```python
from build123d import *

# Parameters (mm, degrees)
BOSS_EXTRUDE1_DEPTH      = 70
BOSS_EXTRUDE1_DEPTH_BACK = 70
SKETCH1_W                = 20
SKETCH1_H                = 10
SKETCH3_W                = 20
SKETCH3_H                = 5
BOSS_EXTRUDE2_DEPTH      = 20
FILLET1_R                = 10
SKETCH4_R                = 2.75
CUT_EXTRUDE1_DEPTH       = 91.863909227
FILLET1_OF_MIRROR1_R     = 10
CHAMFER1_SIZE            = 8.660254038
CHAMFER1_SIZE_2          = 5
SKETCH5_R                = 8.5
CUT_EXTRUDE2_DEPTH       = 5
CUT_EXTRUDE3_DEPTH       = 91.691785736
CUT_EXTRUDE3_DEPTH_BACK  = 91.691785736
SKETCH6_R                = 2


# Some blends are built 0.0001 mm under size
with BuildPart() as part:
    # Sketch1 → Boss-Extrude1 (new, two sides: drawn at the far end of the back side and taken through both)
    with BuildSketch(Plane.XY.offset(-BOSS_EXTRUDE1_DEPTH_BACK)):
        Rectangle(SKETCH1_W, SKETCH1_H)
    extrude(amount=BOSS_EXTRUDE1_DEPTH + BOSS_EXTRUDE1_DEPTH_BACK)

    # Sketch3 → Boss-Extrude2 (add)
    with BuildSketch(Plane(origin=(0, 0, -70), x_dir=(-1, 0, 0), z_dir=(0, 0, -1))):
        Rectangle(SKETCH3_W, SKETCH3_H)
    boss_extrude2 = extrude(amount=BOSS_EXTRUDE2_DEPTH)

    # Fillet1
    fillet1_edges = [part.edges().sort_by_distance(p)[0] for p in [
        (-10, 0, -90),
        (10, 0, -90),
    ]]
    fillet(fillet1_edges, radius=FILLET1_R - 0.0001)  # a hair under: the kernel refuses the full size

    # Sketch4 → Cut-Extrude1 (cut, through all)
    with BuildSketch(Plane(origin=(0, 2.5, 0), x_dir=(1, 0, 0), z_dir=(0, 1, 0))):
        with Locations(Location((0, 80, 0), (0, 0, 270))):
            Circle(SKETCH4_R)
    cut_extrude1 = extrude(amount=-CUT_EXTRUDE1_DEPTH, mode=Mode.SUBTRACT)

    # Mirror1: Boss-Extrude2, Cut-Extrude1 across plane
    add(boss_extrude2.mirror(Plane.XY))
    add(cut_extrude1.mirror(Plane.XY), mode=Mode.SUBTRACT)

    # Fillet1 of Mirror1
    fillet1_of_mirror1_edges = [part.edges().sort_by_distance(p)[0] for p in [
        (-10, 0, 90),
        (10, 0, 90),
    ]]
    fillet(fillet1_of_mirror1_edges, radius=FILLET1_OF_MIRROR1_R - 0.0001)  # a hair under: the kernel refuses the full size

    # Chamfer1
    # the kernel refuses this chamfer: 8.660254038, 5 mm, written as the material it takes off along each edge
    with BuildSketch(Plane(origin=(32.404819853, 5, -70), x_dir=(0, 0.019326765612700594, 0.999813220622208), z_dir=(-1, 0, 0))) as chamfer1_piece_1_section:
        Polygon((CHAMFER1_SIZE * 0.999813220604, -CHAMFER1_SIZE * 0.0193267656124), (-CHAMFER1_SIZE_2 * 0.0193267656127, -CHAMFER1_SIZE_2 * 0.999813220622), (0, 0), align=None)
    chamfer1_piece_1 = extrude(amount=64.809639706, mode=Mode.PRIVATE)
    chamfer1_piece_1 = split(chamfer1_piece_1, bisect_by=Plane(origin=(0, 2.5, -66.539331058), z_dir=(0, 1, 0)), keep=Keep.TOP, mode=Mode.PRIVATE)
    add(chamfer1_piece_1, mode=Mode.SUBTRACT)
    with BuildSketch(Plane(origin=(-32.404819853, -5, -70), x_dir=(0, -0.019326765612700594, 0.999813220622208), z_dir=(1, 0, 0))) as chamfer1_piece_2_section:
        Polygon((CHAMFER1_SIZE * 0.999813220604, -CHAMFER1_SIZE * 0.0193267656124), (-CHAMFER1_SIZE_2 * 0.0193267656127, -CHAMFER1_SIZE_2 * 0.999813220622), (0, 0), align=None)
    chamfer1_piece_2 = extrude(amount=64.809639706, mode=Mode.PRIVATE)
    chamfer1_piece_2 = split(chamfer1_piece_2, bisect_by=Plane(origin=(0, -2.5, -66.539331058), z_dir=(0, -1, 0)), keep=Keep.TOP, mode=Mode.PRIVATE)
    add(chamfer1_piece_2, mode=Mode.SUBTRACT)
    with BuildSketch(Plane(origin=(-32.404819853, -5, 70), x_dir=(0, 0.9983227437537926, 0.05789386240267045), z_dir=(1, 0, 0))) as chamfer1_piece_3_section:
        Polygon((CHAMFER1_SIZE_2 * 0.998322743754, -CHAMFER1_SIZE_2 * 0.0578938624027), (-CHAMFER1_SIZE * 0.0578938624016, -CHAMFER1_SIZE * 0.998322743736), (0, 0), align=None)
    chamfer1_piece_3 = extrude(amount=64.809639706, mode=Mode.PRIVATE)
    chamfer1_piece_3 = split(chamfer1_piece_3, bisect_by=Plane(origin=(0, -2.5, 66.539331058), z_dir=(0, -1, 0)), keep=Keep.TOP, mode=Mode.PRIVATE)
    add(chamfer1_piece_3, mode=Mode.SUBTRACT)
    with BuildSketch(Plane(origin=(32.404819853, 5, 70), x_dir=(0, -0.9983227437537926, 0.05789386240267045), z_dir=(-1, 0, 0))) as chamfer1_piece_4_section:
        Polygon((CHAMFER1_SIZE_2 * 0.998322743754, -CHAMFER1_SIZE_2 * 0.0578938624027), (-CHAMFER1_SIZE * 0.0578938624016, -CHAMFER1_SIZE * 0.998322743736), (0, 0), align=None)
    chamfer1_piece_4 = extrude(amount=64.809639706, mode=Mode.PRIVATE)
    chamfer1_piece_4 = split(chamfer1_piece_4, bisect_by=Plane(origin=(0, 2.5, 66.539331058), z_dir=(0, 1, 0)), keep=Keep.TOP, mode=Mode.PRIVATE)
    add(chamfer1_piece_4, mode=Mode.SUBTRACT)

    # Sketch5 → Cut-Extrude2 (cut)
    with BuildSketch(Plane(origin=(0, 5, 0), x_dir=(1, 0, 0), z_dir=(0, 1, 0))):
        with Locations(Location((0, -46.339745962, 0), (0, 0, 270))):
            Circle(SKETCH5_R)
    extrude(amount=-CUT_EXTRUDE2_DEPTH, mode=Mode.SUBTRACT)

    # Sketch6 → Cut-Extrude3 (cut, two sides: drawn at the far end of the back side and taken through both)
    with BuildSketch(Plane(origin=(0, 0, 0), x_dir=(1, 0, 0), z_dir=(0, 1, 0)).offset(-CUT_EXTRUDE3_DEPTH_BACK)):
        with Locations(Location((0, -46.339745962, 0), (0, 0, 270))):
            Circle(SKETCH6_R)
    extrude(amount=CUT_EXTRUDE3_DEPTH + CUT_EXTRUDE3_DEPTH_BACK, mode=Mode.SUBTRACT)


solid = part.part
```
Can you work these out from the model? Positions are in its coordinate system, mm. A direction names the side the tool comes from. Coordinates: 2 decimals unless noted, no trailing zeros. Loops run counter-clockwise (first coordinate to the right, second up) from the corner with the lowest first, then second, coordinate; pieces in that order, holes last.
Item 1: Suppose I cut it at B-B (z = 63). Please give me the cut outline in (x, y), then the cut area to 3 significant figures.
Answers below:
outline: (-10, -4.04) - (10, -4.04) - (10, 4.04) - (-10, 4.04) - close
area: 162 mm2
Item 2: Which directions (+Z, -Z, +X, -X, +Y, -Y) give clear straight access to the entire face, cutting with the end or side of a thin tool? Please do faces 1 (the face through (0, 2.5, -75)), 2 (the face through (0, 2.5, 75)), 3 (the face through (0, 0, 44)).
Answers below:
face 1: -Z, +X, -X, +Y
face 2: +Z, +X, -X, +Y
face 3: +Y
Item 3: Suppose I cut it at A-A (x = 5). Please give me the cut outline in (y, z), then the cut area to 3 significant figures.
Answers below:
outline: (-5, -61.34) - (-2.5, -65.67) - (-2.5, -88.66) - (2.5, -88.66) - (2.5, -65.67) - (5, -61.34) - (5, 39.47) - (0, 39.47) - (0, 53.21) - (5, 53.21) - (5, 61.34) - (2.5, 65.67) - (2.5, 88.66) - (-2.5, 88.66) - (-2.5, 65.67) - (-5, 61.34) - close
area: 1,450 mm2
Item 4: If we mould it in two halves opening along X, with no side actions, what happens to faces 4 (the face through (0, -2.5, -75)), 5 (the face through (-10, 0, -1)), 6 (the face through (10, 0, -1)), 7 (the face through (0.121, 0.035, -82.747))? For each: released by +X, released by -X, zero draft, split by the parting line, or undercut.
Answers below:
face 4: zero draft
face 5: released by -X
face 6: released by +X
face 7: undercut
Item 5: Please list where these lines run through material, in increasing order: L1, parallel to X at y = -0.2, z = 80; L2, parallel to Y at x = 8, z = -75; L3, parallel to Z at x = -6, y = 4.25.
Answers below:
L1: x = -10 to -2.75, 2.75 to 10
L2: y = -2.5 to 2.5
L3: z = -62.64 to 40.32, 52.36 to 62.64
Item 6: I'm going to push flat-ended pins straight in: pin 1 (6 mm diameter, centred on x = -4.5, z = -75, fed in from +Y); pin 2 (4.5 mm diameter, centred on x = 0, z = -80, fed in from +Y); pin 3 (10 mm diameter, centred on x = -1, z = 70, fed in from -Y); pin 4 (5 mm diameter, centred on x = -1.5, z = 45, fed in from +Y). Where does each tip first touch, or does it pass through?
Answers below:
pin 1: stops at y = 2.5
pin 2: passes through
pin 3: stops at y = -2.89
pin 4: stops at y = 0
